For this review, take the finished solid that the model builds, in its own axes (mm). A direction names the side the tool comes from. Give positions to 0.01 mm unless a question says otherwise; leave off trailing zeros. Write each loop counter-clockwise with the first axis right and the second up, starting at its lowest first coordinate (ties: lowest second). Pieces come first, ordered by that corner, then holes.
from build123d import *

# Parameters (mm, degrees)
SKETCH1_W           = 85
SKETCH1_H           = 56
SKETCH1_R           = 1.25
BOSS_EXTRUDE1_DEPTH = 4
SKETCH2_R           = 3
SKETCH2_R_2         = 1.25
BOSS_EXTRUDE2_DEPTH = 4
FILLET1_R           = 3
BOSS_EXTRUDE4_DEPTH = 4
SKETCH3_R           = 2.5
CUT_EXTRUDE1_DEPTH  = 59.5
FILLET2_R           = 10


with BuildPart() as part:
    # Sketch1 → Boss-Extrude1 (new body)
    with BuildSketch(Plane(origin=(0, 0, 0), x_dir=(1, 0, 0), z_dir=(0, 1, 0))):
        Rectangle(SKETCH1_W, SKETCH1_H)
        with Locations(Location((-39, 24.5, 0), (0, 0, 270))):
            Circle(SKETCH1_R, mode=Mode.SUBTRACT)
        with Locations(Location((-39, -24.5, 0), (0, 0, 270))):
            Circle(SKETCH1_R, mode=Mode.SUBTRACT)
        with Locations(Location((19, 24.5, 0), (0, 0, 270))):
            Circle(SKETCH1_R, mode=Mode.SUBTRACT)
        with Locations(Location((19, -24.5, 0), (0, 0, 270))):
            Circle(SKETCH1_R, mode=Mode.SUBTRACT)
    extrude(amount=BOSS_EXTRUDE1_DEPTH)

    # Sketch2 → Boss-Extrude2 (add)
    # profile 1 of 4: a face of its own
    with BuildSketch(Plane(origin=(0, 4, 0), x_dir=(1, 0, 0), z_dir=(0, 1, 0))):
        with Locations(Location((-39, 24.5, 0), (0, 0, 270))):
            Circle(SKETCH2_R)
        with Locations(Location((-39, 24.5, 0), (0, 0, 270))):
            Circle(SKETCH2_R_2, mode=Mode.SUBTRACT)
    # profile 2 of 4: a face of its own
    with BuildSketch(Plane(origin=(0, 4, 0), x_dir=(1, 0, 0), z_dir=(0, 1, 0))):
        with Locations(Location((19, 24.5, 0), (0, 0, 270))):
            Circle(SKETCH2_R)
        with Locations(Location((19, 24.5, 0), (0, 0, 270))):
            Circle(SKETCH2_R_2, mode=Mode.SUBTRACT)
    # profile 3 of 4: a face of its own
    with BuildSketch(Plane(origin=(0, 4, 0), x_dir=(1, 0, 0), z_dir=(0, 1, 0))):
        with Locations(Location((19, -24.5, 0), (0, 0, 270))):
            Circle(SKETCH2_R)
        with Locations(Location((19, -24.5, 0), (0, 0, 270))):
            Circle(SKETCH2_R_2, mode=Mode.SUBTRACT)
    # profile 4 of 4: a face of its own
    with BuildSketch(Plane(origin=(0, 4, 0), x_dir=(1, 0, 0), z_dir=(0, 1, 0))):
        with Locations(Location((-39, -24.5, 0), (0, 0, 270))):
            Circle(SKETCH2_R)
        with Locations(Location((-39, -24.5, 0), (0, 0, 270))):
            Circle(SKETCH2_R_2, mode=Mode.SUBTRACT)
    extrude(amount=BOSS_EXTRUDE2_DEPTH)

    # Fillet1
    fillet1_edges = [part.edges().sort_by_distance(p)[0] for p in [
        (-42.5, 2, 28),
        (-42.5, 2, -28),
        (42.5, 2, -28),
        (42.5, 2, 28),
    ]]
    fillet(fillet1_edges, radius=FILLET1_R)

    # Sketch5 → Boss-Extrude4 (add)
    with BuildSketch(Plane(origin=(0, 0, 0), x_dir=(1, 0, 0), z_dir=(0, 1, 0))):
        Polygon((-40, -30), (-17, -10), (-17, 10), (-40, 30), (-40, 40), (-30, 40), (-10, 17), (10, 17), (30, 40), (40, 40), (40, 30), (17, 10), (17, -10), (40, -30), (40, -40), (30, -40), (10, -17), (-10, -17), (-30, -40), (-40, -40), align=None)
    extrude(amount=BOSS_EXTRUDE4_DEPTH)

    # Sketch3 → Cut-Extrude1 (cut, through all)
    with BuildSketch(Plane(origin=(0, 4, 0), x_dir=(1, 0, 0), z_dir=(0, 1, 0))):
        with Locations(Location((-31.819805153, 31.819805153, 0), (0, 0, 270))):
            Circle(SKETCH3_R)
        with Locations(Location((-24.748737342, 24.748737342, 0), (0, 0, 270))):
            Circle(SKETCH3_R)
        with Locations(Location((31.819805153, 31.819805153, 0), (0, 0, 270))):
            Circle(SKETCH3_R)
        with Locations(Location((24.748737342, 24.748737342, 0), (0, 0, 270))):
            Circle(SKETCH3_R)
        with Locations(Location((24.748737342, -24.748737342, 0), (0, 0, 270))):
            Circle(SKETCH3_R)
        with Locations(Location((31.819805153, -31.819805153, 0), (0, 0, 270))):
            Circle(SKETCH3_R)
        with Locations(Location((-31.819805153, -31.819805153, 0), (0, 0, 270))):
            Circle(SKETCH3_R)
        with Locations(Location((-24.748737342, -24.748737342, 0), (0, 0, 270))):
            Circle(SKETCH3_R)
    extrude(amount=-CUT_EXTRUDE1_DEPTH, mode=Mode.SUBTRACT)

    # Fillet2
    # the kernel refuses this fillet: 10 mm, written as the material it takes off along each edge
    with BuildSketch(Plane(origin=(-40, -10.951097141, -30), x_dir=(0.7546055221635131, 0, 0.6561787149247771), z_dir=(0, 1, 0))) as fillet2_piece_1_section:
        with BuildLine():
            CenterArc((4.671704482, 9.8672905), FILLET2_R, 221.009086902, 39.646111147)
            Line((-2.87435074, 3.305503351), (-3.025271844, 3.174267608))
            Line((-3.025271844, 3.174267608), (-0.150921104, -0.131235743))
            Line((-0.150921104, -0.131235743), (0, -0.2))
            ThreePointArc((0, -0.2), (1.523975065, -0.2), (3.015475044, -0.19734581))
            Line((3.015475044, -0.19734581), (3.047950131, 0))
        make_face()
    fillet2_piece_1 = extrude(amount=25.902194282, mode=Mode.PRIVATE)
    fillet2_piece_1 = split(fillet2_piece_1, bisect_by=Plane(origin=(-39.506364614, 2, -28), z_dir=(0, 0, -1)), keep=Keep.TOP, mode=Mode.PRIVATE)
    add(fillet2_piece_1, mode=Mode.SUBTRACT)
    with BuildSketch(Plane(origin=(-40, -25, -40), x_dir=(0, 0, 1), z_dir=(0, 1, 0)), Plane(origin=(40, -25, -40), x_dir=(-1, 0, 0), z_dir=(0, 1, 0))) as fillet2_piece_2:
        with BuildLine():
            CenterArc((FILLET2_R, FILLET2_R), FILLET2_R, 180, 90)
            Line((0, FILLET2_R), (-FILLET2_R * 0.02, FILLET2_R))
            Line((-FILLET2_R * 0.02, FILLET2_R), (-FILLET2_R * 0.02, -FILLET2_R * 0.02))
            Line((-FILLET2_R * 0.02, -FILLET2_R * 0.02), (FILLET2_R, -FILLET2_R * 0.02))
            Line((FILLET2_R, -FILLET2_R * 0.02), (FILLET2_R, 0))
        make_face()
    extrude(amount=54, mode=Mode.SUBTRACT)
    with BuildSketch(Plane(origin=(-30, -11.390762292, -40), x_dir=(-1, 0, 0), z_dir=(0, 1, 0)), Plane(origin=(30, -11.390762292, -40), x_dir=(-0.6561787149247741, 0, 0.7546055221635154), z_dir=(0, 1, 0))) as fillet2_piece_3:
        with BuildLine():
            CenterArc((FILLET2_R * 0.455630491663, FILLET2_R), FILLET2_R, 221.009086902, 48.990913098)
            Line((-FILLET2_R * 0.2989750305, FILLET2_R * 0.343821285075), (-FILLET2_R * 0.314067140943, FILLET2_R * 0.330697710777))
            Line((-FILLET2_R * 0.314067140943, FILLET2_R * 0.330697710777), (-FILLET2_R * 0.00911260983327, -FILLET2_R * 0.02))
            Line((-FILLET2_R * 0.00911260983327, -FILLET2_R * 0.02), (FILLET2_R * 0.455630491663, -FILLET2_R * 0.02))
            Line((FILLET2_R * 0.455630491663, -FILLET2_R * 0.02), (FILLET2_R * 0.455630491663, 0))
        make_face()
    extrude(amount=26.781524583, mode=Mode.SUBTRACT)
    with BuildSketch(Plane(origin=(40, -10.951097141, -30), x_dir=(0, 0, -1), z_dir=(0, 1, 0))) as fillet2_piece_4_section:
        with BuildLine():
            CenterArc((4.380438856, 10), FILLET2_R, 230.353888853, 39.646111147)
            Line((-2, 2.3), (-2.127608777, 2.146))
            ThreePointArc((-2.127608777, 2.146), (-1.150921104, 1.018764257), (-0.150921104, -0.131235743))
            Line((-0.150921104, -0.131235743), (0, -0.2))
            Line((0, -0.2), (4.380438856, -0.2))
            Line((4.380438856, -0.2), (4.380438856, 0))
        make_face()
    fillet2_piece_4 = extrude(amount=25.902194282, mode=Mode.PRIVATE)
    fillet2_piece_4 = split(fillet2_piece_4, bisect_by=Plane(origin=(39.506364614, 2, -28), z_dir=(0, 0, -1)), keep=Keep.TOP, mode=Mode.PRIVATE)
    add(fillet2_piece_4, mode=Mode.SUBTRACT)
    with BuildSketch(Plane(origin=(40, -10.951097141, 30), x_dir=(0, 0, 1), z_dir=(0, 1, 0))) as fillet2_piece_5_section:
        with BuildLine():
            CenterArc((4.380438856, -10), FILLET2_R, 90, 39.646111147)
            Line((-2, -2.3), (-2.127608777, -2.146))
            ThreePointArc((-2.127608777, -2.146), (-1.150921104, -1.018764257), (-0.150921104, 0.131235743))
            Line((-0.150921104, 0.131235743), (0, 0.2))
            Line((0, 0.2), (4.380438856, 0.2))
            Line((4.380438856, 0.2), (4.380438856, 0))
        make_face()
    fillet2_piece_5 = extrude(amount=25.902194282, mode=Mode.PRIVATE)
    fillet2_piece_5 = split(fillet2_piece_5, bisect_by=Plane(origin=(39.506364614, 2, 28), z_dir=(0, 0, 1)), keep=Keep.TOP, mode=Mode.PRIVATE)
    add(fillet2_piece_5, mode=Mode.SUBTRACT)
    with BuildSketch(Plane(origin=(40, -25, 40), x_dir=(-1, 0, 0), z_dir=(0, 1, 0)), Plane(origin=(-40, -25, 40), x_dir=(0, 0, -1), z_dir=(0, 1, 0))) as fillet2_piece_6:
        with BuildLine():
            CenterArc((FILLET2_R, -FILLET2_R), FILLET2_R, 90, 90)
            Line((0, -FILLET2_R), (-FILLET2_R * 0.02, -FILLET2_R))
            Line((-FILLET2_R * 0.02, -FILLET2_R), (-FILLET2_R * 0.02, FILLET2_R * 0.02))
            Line((-FILLET2_R * 0.02, FILLET2_R * 0.02), (FILLET2_R, FILLET2_R * 0.02))
            Line((FILLET2_R, FILLET2_R * 0.02), (FILLET2_R, 0))
        make_face()
    extrude(amount=54, mode=Mode.SUBTRACT)
    with BuildSketch(Plane(origin=(30, -11.390762292, 40), x_dir=(-0.6561787149247873, 0, -0.7546055221635042), z_dir=(0, 1, 0)), Plane(origin=(-30, -11.390762292, 40), x_dir=(-1, 0, 0), z_dir=(0, 1, 0))) as fillet2_piece_7:
        with BuildLine():
            CenterArc((FILLET2_R * 0.455630491663, -FILLET2_R), FILLET2_R, 90, 48.990913098)
            Line((-FILLET2_R * 0.2989750305, -FILLET2_R * 0.343821285075), (-FILLET2_R * 0.314067140943, -FILLET2_R * 0.330697710777))
            Line((-FILLET2_R * 0.314067140943, -FILLET2_R * 0.330697710777), (-FILLET2_R * 0.00911260983327, FILLET2_R * 0.02))
            Line((-FILLET2_R * 0.00911260983327, FILLET2_R * 0.02), (FILLET2_R * 0.455630491663, FILLET2_R * 0.02))
            Line((FILLET2_R * 0.455630491663, FILLET2_R * 0.02), (FILLET2_R * 0.455630491663, 0))
        make_face()
    extrude(amount=26.781524583, mode=Mode.SUBTRACT)
    with BuildSketch(Plane(origin=(-40, -10.951097141, 30), x_dir=(0.7546055221635047, 0, -0.6561787149247865), z_dir=(0, 1, 0))) as fillet2_piece_8_section:
        with BuildLine():
            CenterArc((4.671704482, -9.8672905), FILLET2_R, 99.344801951, 39.646111147)
            Line((-2.87435074, -3.305503351), (-3.025271844, -3.174267608))
            Line((-3.025271844, -3.174267608), (-0.150921104, 0.131235743))
            Line((-0.150921104, 0.131235743), (0, 0.2))
            ThreePointArc((0, 0.2), (1.523975065, 0.2), (3.015475044, 0.19734581))
            Line((3.015475044, 0.19734581), (3.047950131, 0))
        make_face()
    fillet2_piece_8 = extrude(amount=25.902194282, mode=Mode.PRIVATE)
    fillet2_piece_8 = split(fillet2_piece_8, bisect_by=Plane(origin=(-39.506364614, 2, 28), z_dir=(0, 0, 1)), keep=Keep.TOP, mode=Mode.PRIVATE)
    add(fillet2_piece_8, mode=Mode.SUBTRACT)


solid = part.part
(1) Clearance check with flat-ended pins moving along their axes: pin 1 Ø0.5 at (x, y) = (39, 1.5) entering from -Z; pin 2 Ø4.5 at (x, z) = (31.82, -31.82) entering from -Y; pin 3 Ø10 at (x, z) = (-2, -14) entering from +Y; pin 4 Ø1.4 at (x, y) = (38.5, 2) entering from +Z. State where each tip first meets the part, or that it passes through.
(2) Tool access review of faces 1 (the cylindrical face through (17.2, 6, 22.1)), 2 (the flat face through (0, 2, -28)), 3 (the cylindrical face through (-29.432, 1.972, 38.587)), 4 (the cylindrical face through (23.791, 2.028, 27.058)): name each direction out of +Z, -Z, +X, -X, +Y, -Y from which nothing blocks a thin tool from reaching the whole face with its end or side.
(3) The part is to be moulded in two halves that separate along Z. For faces 5 (the flat face through (-39, 8, 26)), 6 (the flat face through (19, 4, 24)), 7 (the flat face through (-23.236, 1.972, 32.221)), say which applies: +Z half, -Z half, draft (parallel to the pull), parting line (faces both ways), or undercut.
(4) We need section A-A (y = 7). Write out the cut boundary in (x, z), and give its area (3 significant figures).
(5) We need section B-B (x = 11). Write out the cut boundary in (y, z), and give its area (3 significant figures).
(6) For L1, parallel to X at y = 7.05, z = 24.5; L2, parallel to Z at x = 19, y = 6.75; L3, parallel to X at y = 3.25, z = -32, list the stretches that pass through material, from the lowest coordinate up.
(7) We need section C-C (z = -4). Write out the cut boundary in (x, y), and give its area (3 significant figures).
(8) We need section D-D (y = 1.25). Count the separate pieces of the cut face and the enclosed holes in it, and give its area (3 significant figures).
The answers:
1. pin 1: stops at z = -34.84
1. pin 2: passes through
1. pin 3: stops at y = 4
1. pin 4: stops at z = 36.26
2. face 1: +Y
2. face 2: -Z, +Y, -Y
2. face 3: +Z, +Y, -Y
2. face 4: +Y, -Y
3. face 5: draft
3. face 6: undercut
3. face 7: +Z half
4. outline: circle Ø6 at (-39, -24.5); circle Ø6 at (-39, 24.5); circle Ø6 at (19, -24.5); circle Ø6 at (19, 24.5); hole circle Ø2.5 at (-39, -24.5); hole circle Ø2.5 at (-39, 24.5); hole circle Ø2.5 at (19, -24.5); hole circle Ø2.5 at (19, 24.5)
4. area: 93.5 mm2
5. outline: (0, -28) - (4, -28) - (4, 28) - (0, 28) - close
5. area: 224 mm2
6. L1: x = -42 to -40.25, -37.75 to -36, 16 to 17.75, 20.25 to 22
6. L2: z = -27.5 to -25.75, -23.25 to -21.5, 21.5 to 23.25, 25.75 to 27.5
6. L3: x = -39.71 to -34.31, -29.33 to -23.04, 23.04 to 29.33, 34.31 to 39.71
7. outline: (-42.5, 0) - (42.5, 0) - (42.5, 4) - (-42.5, 4) - close
7. area: 340 mm2
8. separate pieces: 1
8. enclosed holes: 10
8. area: 5,200 mm2
